Part print with two shaded views. Sizes in mm from the minimum x, y, z corner. A direction names the side the tool comes from. Round coordinates to 2 decimals unless told otherwise and drop trailing zeros. Order: outer loops, then holes, each group sorted by start corner. A loop starts at its lowest first (then second) coordinate and runs counter-clockwise, first axis right, second up. Notation, with made-up numbers: (48, -31) -> (100, -31) arc R27 cw to (100, 6) -> close; hole circle Ø7 at (83, 58.25). An arc over 180 degrees is marked (long way). Use a Markdown table: item, result. Add a question column.
Item 1: Probe L1, parallel to Z at x = 66, y = 35; L2, parallel to Y at x = 9.5, z = 42.5; L3, parallel to X at y = 9, z = 48. List the from-to ranges inside material, lowest first.
Item 2: Slice it at B-B, the plane y = 35. Give the cut face in (x, z).
Item 3: 3-axis set-ups, long thin cutter, end or side, ignore diameter. For the marked faces 1 and 2: which of +Z, -Z, +X, -X, +Y, -Y reach the whole face in a straight line?
Item 4: Pin check, flat tips, straight feed: pin 1 (2 mm diameter, centred on x = 17.5, z = 95, fed in from +Y); pin 2 (5 mm diameter, centred on y = 40, z = 35, fed in from -X). Stop position of each tip, or through.
Item 5: Slice it at A-A, the plane z = 115. Give the cut face in (x, y).
Item 6: Slice it at C-C, the plane y = 22. Give the cut face in (x, z), plus the area to 3 significant figures.
Item 7: Slice it at D-D, the plane z = 66. Give the cut face in (x, y), plus the area to 3 significant figures.
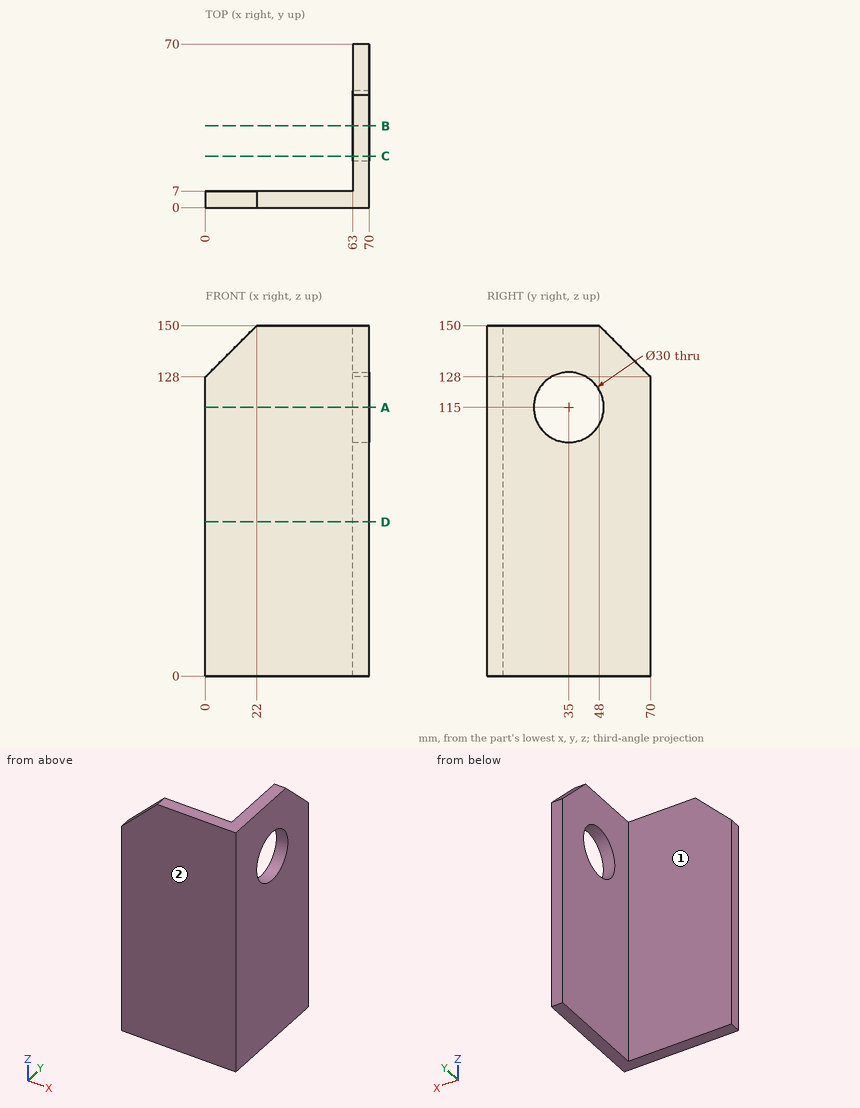
Check sheet entries:
| question | item | result |
|---|---|---|
| 1 | L1 | 0 to 100, 130 to 150 |
| 1 | L2 | 0 to 7 |
| 1 | L3 | 63 to 70 |
| 2 | outline | (63, 0) -> (70, 0) -> (70, 100) -> (63, 100) -> close; (63, 130) -> (70, 130) -> (70, 150) -> (63, 150) -> close |
| 3 | face 1 | +Z, -Z, -X, +Y |
| 3 | face 2 | +Z, -Z, +X, -X, -Y |
| 4 | pin 1 | y = 7 |
| 4 | pin 2 | x = 63 |
| 5 | outline | (0, 0) -> (70, 0) -> (70, 20) -> (63, 20) -> (63, 7) -> (0, 7) -> close; (63, 50) -> (70, 50) -> (70, 70) -> (63, 70) -> close |
| 6 | outline | (63, 0) -> (70, 0) -> (70, 107.52) -> (63, 107.52) -> close; (63, 122.48) -> (70, 122.48) -> (70, 150) -> (63, 150) -> close |
| 6 | area | 945 mm2 |
| 7 | outline | (0, 0) -> (70, 0) -> (70, 70) -> (63, 70) -> (63, 7) -> (0, 7) -> close |
| 7 | area | 931 mm2 |
